```python
from build123d import *
from OCP.BRepFilletAPI import BRepFilletAPI_MakeChamfer

# Parameters (mm, degrees)
RESSALTO_EXTRUS_O1_DEPTH = 9
ESBO_O2_W                = 9
ESBO_O2_H                = 9
ESBO_O2_W_2              = 6.3
ESBO_O2_H_2              = 6.3
CORTE_EXTRUS_O1_DEPTH    = 8
ESBO_O3_R                = 2.25
CORTE_EXTRUS_O2_DEPTH    = 29.390139133
CHANFRO2_SIZE            = 2
CHANFRO2_SIZE_2          = 1.35


with BuildPart() as part:
    # Esboço1 → Ressalto-extrusão1 (new body)
    with BuildSketch(Plane(origin=(0, 0, 0), x_dir=(1, 0, 0), z_dir=(0, 1, 0))):
        Polygon((0, 0), (25, 0), (25, 5), (17, 5), (17, 15), (8, 15), (8, 5), (0, 5), align=None)
    extrude(amount=RESSALTO_EXTRUS_O1_DEPTH)

    # Esboço2 → Corte-extrusão1 (cut)
    with BuildSketch(Plane(origin=(0, 0, -15), x_dir=(-1, 0, 0), z_dir=(0, 0, -1))):
        with Locations((-12.5, 4.5)):
            Rectangle(ESBO_O2_W, ESBO_O2_H)
        with Locations((-12.5, 4.5)):
            Rectangle(ESBO_O2_W_2, ESBO_O2_H_2, mode=Mode.SUBTRACT)
    extrude(amount=-CORTE_EXTRUS_O1_DEPTH, mode=Mode.SUBTRACT)

    # Esboço3 → Corte-extrusão2 (cut, through all)
    with BuildSketch(Plane(origin=(0, 0, -5), x_dir=(-1, 0, 0), z_dir=(0, 0, -1))):
        with Locations((-4, 4.5)):
            Circle(ESBO_O3_R)
        with Locations((-21, 4.5)):
            Circle(ESBO_O3_R)
    extrude(amount=-CORTE_EXTRUS_O2_DEPTH, mode=Mode.SUBTRACT)

    # Chanfro2
    chanfro2_edges_1 = [part.edges().sort_by_distance(p)[0] for p in [
        (8, 4.5, -7),
    ]]
    chanfro2_side_1 = [part.faces().sort_by_distance(p)[0] for p in [
        (8, 4.5, -6.973),
    ]]
    chanfro2_edges_2 = [part.edges().sort_by_distance(p)[0] for p in [
        (17, 4.5, -7),
    ]]
    chanfro2_side_2 = [part.faces().sort_by_distance(p)[0] for p in [
        (16.973, 4.5, -7),
    ]]
    chanfro2 = BRepFilletAPI_MakeChamfer(part.part.solid().wrapped)
    for e in chanfro2_edges_1:
        chanfro2.Add(CHANFRO2_SIZE - 0.0001, CHANFRO2_SIZE_2 - 0.0001, e.wrapped, chanfro2_side_1[0].wrapped)
    for e in chanfro2_edges_2:
        chanfro2.Add(CHANFRO2_SIZE_2 - 0.0001, CHANFRO2_SIZE - 0.0001, e.wrapped, chanfro2_side_2[0].wrapped)
    add(Compound.cast(chanfro2.Shape()), mode=Mode.REPLACE)  # a hair under: the kernel refuses the full size


solid = part.part
```
Work out the finished part from the listing and answer in its coordinate system (mm). A direction names the side the tool comes from. Give positions to 0.01 mm unless a question says otherwise; leave off trailing zeros. Write each loop counter-clockwise with the first axis right and the second up, starting at its lowest first coordinate (ties: lowest second). Pieces come first, ordered by that corner, then holes. Notation, with made-up numbers: (60.25, 87.25) - (88.25, 87.25) arc R17 cw to (88.25, 99.25) - close; hole circle Ø1 at (84, -25). An arc over 180 degrees is marked (long way). Use one line per item in the form item = value.
1. For faces 4 (the face through (13, 7.65, -11)), 5 (the face through (13, 1.35, -11)), 6 (the face through (9.35, 4, -11)), 7 (the face through (13, 1, -7)), 8 (the face through (22, 2, -5)), determine the directions among +Z, -Z, +X, -X, +Y, -Y from which every point of the face is accessible in a straight line to the end or side of a thin tool.
Filled in:
face_4 = -Z, +X, -X, +Y
face_5 = -Z, +X, -X, -Y
face_6 = -Z, -X, +Y, -Y
face_7 = -Z, +X, -X
face_8 = -Z, +X, +Y, -Y
2. A cutting plane is placed at B-B (y = 4.5). State how many separate pieces and enclosed holes the cut face has, and give its area (3 significant figures).
Filled in:
separate_pieces = 3
enclosed_holes = 0
area = 146 mm^2
3. Determine the mould class of faces 1 (the face through (18.854, 5.176, -2.535)), 2 (the face through (12, 0, -3)), 3 (the face through (15.65, 4, -11)) for opening direction X: released by +X, released by -X, zero draft, split by the parting line, or undercut.
Filled in:
face_1 = undercut
face_2 = zero draft
face_3 = released by +X
4. Consider L1, parallel to Y at x = 4, z = -2.05; L2, parallel to Z at x = 19.75, y = 7; L3, parallel to X at y = 6, z = -12.25. Determine where each line is inside the solid, lowest interval first.
Filled in:
L1 = 0 to 2.25, 6.75 to 9
L2 = -5 to 0
L3 = 9.35 to 15.65
5. A cutting plane is placed at A-A (x = 4). Write down the section's boundary in (y, z), and give its area (3 significant figures).
Filled in:
outline = (0, -5) - (2.25, -5) - (2.25, 0) - (0, 0) - close; (6.75, -5) - (9, -5) - (9, 0) - (6.75, 0) - close
area = 22.5 mm^2
6. A cutting plane is placed at D-D (x = 18). Write down the section's boundary in (y, z), and give its area (3 significant figures).
Filled in:
outline = (0, -5) - (9, -5) - (9, 0) - (0, 0) - close
area = 45.0 mm^2
7. Each of these flat-tipped pins is pushed along its axis until it touches: pin 1 Ø2.5 at (x, y) = (5.5, 4.5) entering from -Z; pin 2 Ø2 at (x, z) = (9.5, -5) entering from -Y; pin 3 Ø6 at (x, z) = (17.5, -13) entering from +Y; pin 4 Ø1.5 at (y, z) = (7, -7) entering from -X. Where does it stop, or does it pass through?
Filled in:
pin_1 = -5
pin_2 = 0
pin_3 = 7.65
pin_4 = 8.84
